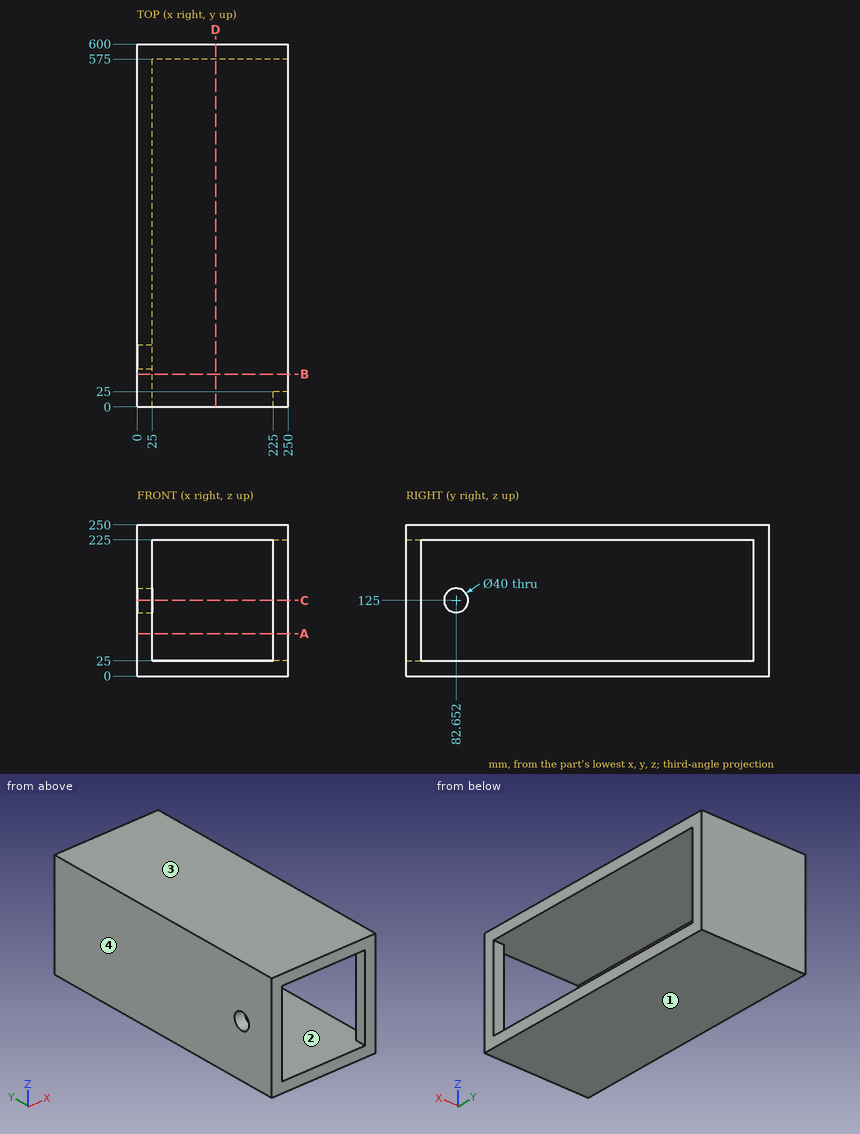
Source: three-view drawing plus pictorial views. Frame: mm from the lowest corner of the part. Give positions to 0.01 mm unless a question says otherwise; leave off trailing zeros. Order: outer loops, then holes, each group sorted by start corner. A loop starts at its lowest first (then second) coordinate and runs counter-clockwise, first axis right, second up. Notation, with made-up numbers: M -20,78.25 L -12,78.25 A22 cw -12,102.25 Z; hole C 69.5,85.25 d5. An arc over 180 degrees is marked long. Return JSON: item names as keys, results as strings.
1) Mould query, pull axis Z, two halves, no side actions, for the marked faces 1, 2, 3 and 4. Classes: released by +Z, released by -Z, zero draft, split by the parting line, or undercut.
Taken from the geometry:
{"face 1": "released by -Z", "face 2": "undercut", "face 3": "released by +Z", "face 4": "zero draft"}
2) Line query: L1, parallel to Z at x = 223, y = 359.5; L2, parallel to Y at x = 193.5, z = 198.5; L3, parallel to X at y = 412.5, z = 220.5. Output: solid intervals per line, ascending. Write a range as [from, to].
Taken from the geometry:
{"L1": "z = [0, 25], [225, 250]", "L2": "y = [575, 600]", "L3": "x = [0, 25]"}
3) Section query C-C on z = 125. Output: boundary loops of the cut face in (x, y), and give its area (4 significant figures).
Taken from the geometry:
{"outline": "M 0,0 L 25,0 L 25,62.65 L 0,62.65 Z; M 0,102.65 L 25,102.65 L 25,575 L 250,575 L 250,600 L 0,600 Z; M 225,0 L 250,0 L 250,25 L 225,25 Z", "area": "20,250 mm2"}
4) Contact query for flat-ended pins moving along their axis: pin 1 (8 mm diameter, centred on x = 219, z = 140.5, fed in from -Y); pin 2 (24 mm diameter, centred on y = 82.65, z = 125, fed in from -X); pin 3 (12.5 mm diameter, centred on y = 16, z = 92.5, fed in from -X). Output: stop coordinate, or through.
Taken from the geometry:
{"pin 1": "stops at y = 575", "pin 2": "passes through", "pin 3": "stops at x = 0"}
5) Section query A-A on z = 70. Output: boundary loops of the cut face in (x, y).
Taken from the geometry:
{"outline": "M 0,0 L 25,0 L 25,575 L 250,575 L 250,600 L 0,600 Z; M 225,0 L 250,0 L 250,25 L 225,25 Z"}
6) Section query D-D on x = 130. Output: boundary loops of the cut face in (y, z), and give its area (3 significant figures).
Taken from the geometry:
{"outline": "M 0,0 L 600,0 L 600,250 L 0,250 L 0,225 L 575,225 L 575,25 L 0,25 Z", "area": "35,000 mm2"}
7) Section query B-B on y = 54. Output: boundary loops of the cut face in (x, z).
Taken from the geometry:
{"outline": "M 0,0 L 250,0 L 250,25 L 25,25 L 25,225 L 250,225 L 250,250 L 0,250 Z"}
